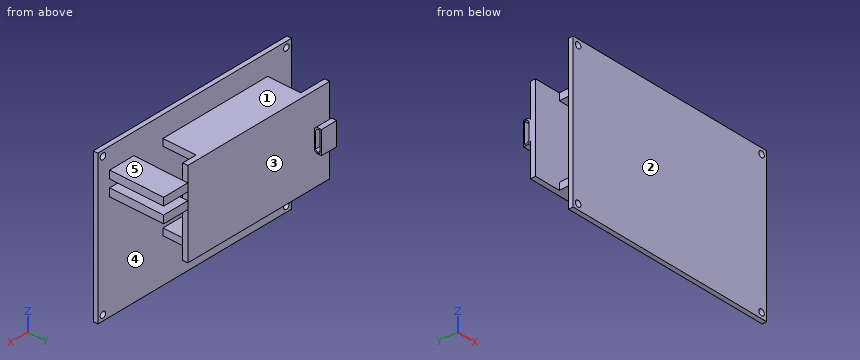
Autodesk Inventor part; units mm, degrees
ref_plane "YZ Plane" through (0, 0, 0) normal (1, 0, 0) x (0, 1, 0)
ref_plane "XZ Plane" through (0, 0, 0) normal (0, 1, 0) x (-1, 0, 0)
ref_plane "XY Plane" through (0, 0, 0) normal (0, 0, 1) x (1, 0, 0)
sketch "Sketch1" plane through (0, 0, 0) normal (0, 1, 0) x (-1, 0, 0)
  line L0 (-35, 25) -> (35, 25)
  line L1 (35, 25) -> (35, -25)
  line L2 (35, -25) -> (-35, -25)
  line L3 (-35, -25) -> (-35, 25)
  line L4 (-35, 25) -> (35, -25) construction
  line L5 (35, 25) -> (-35, -25) construction
  point P0 (0, 0)
  dimension "d0" = 70
  dimension "d1" = 50
extrude "Extrusion1" add sketch "Sketch1" along normal blind 1.5
sketch "Sketch4" plane through (0, 1.5, 0) normal (0, 1, 0) x (1, 0, 0)
  line L0 (16.25, 10.5) -> (-35, 10.5)
  line L1 (-35, 10.5) -> (-35, -18)
  line L2 (-35, -18) -> (16.25, -18)
  line L3 (16.25, -18) -> (16.25, 10.5)
  line L4 (16.25, 10.5) -> (-35, -18) construction
  line L5 (-35, 10.5) -> (16.25, -18) construction
  line L6 (-35, -25) -> (35, -25)
  line L7 (-35, 25) -> (-35, -25)
  dimension "d10" = 51.25
  dimension "d11" = 28.5
  dimension "d12" = 7
extrude "Extrusion3" add sketch "Sketch4" along normal blind 12.7
sketch "Sketch5" plane through (0, 1.5, 0) normal (0, 1, 0) x (1, 0, 0)
  line L0 (30.74, -15.4) -> (22, -15.4)
  line L1 (22, -15.4) -> (22, -18)
  line L2 (22, -18) -> (30.74, -18)
  line L3 (30.74, -18) -> (30.74, -15.4)
  line L4 (30.74, -15.4) -> (22, -18) construction
  line L5 (22, -15.4) -> (30.74, -18) construction
  line L6 (16.25, -18) -> (16.25, 10.5)
  line L7 (-35, -18) -> (16.25, -18)
  line L8 (30.74, -10.2) -> (22, -10.2)
  line L9 (22, -10.2) -> (22, -12.8)
  line L10 (22, -12.8) -> (30.74, -12.8)
  line L11 (30.74, -12.8) -> (30.74, -10.2)
  line L12 (30.74, -10.2) -> (22, -12.8) construction
  line L13 (22, -10.2) -> (30.74, -12.8) construction
  point P0 (0, 0)
  point P1 (26.37, -16.7)
  point P2 (22, -16.7)
  point P3 (26.37, -11.5)
  point P4 (22, -11.5)
  dimension "d15" = 5.75
  dimension "d16" = 8.74
  dimension "d17" = 2.6
  dimension "d18" = 8.74
  dimension "d19" = 2.6
  dimension "d20" = 2.6
extrude "Extrusion4" add sketch "Sketch5" along normal blind 18
sketch "Sketch6" plane through (-35, 0, -25) normal (-1, 0, 0) x (0, 0, 1)
  line L0 (24.91, 16.55) -> (32.59, 16.55)
  line L1 (32.59, 16.55) -> (32.59, 14.9)
  line L2 (31.89, 14.2) -> (25.61, 14.2)
  line L3 (24.91, 14.9) -> (24.91, 16.55)
  line L4 (24.91, 16.55) -> (32.59, 14.2) construction
  line L5 (32.59, 16.55) -> (24.91, 14.2) construction
  line L6 (43, 1.5) -> (50, 1.5)
  line L7 (43, 1.5) -> (43, 14.2)
  line L8 (14.5, 1.5) -> (14.5, 14.2)
  line L9 (32.18, 16.14) -> (25.32, 16.14)
  line L10 (25.32, 16.14) -> (25.32, 15.31)
  line L11 (26.02, 14.61) -> (31.48, 14.61)
  line L12 (32.18, 15.31) -> (32.18, 16.14)
  line L13 (14.5, 14.2) -> (43, 14.2)
  line L14 (25.32, 15.31) -> (26.02, 14.61)
  line L15 (32.18, 15.31) -> (31.48, 14.61)
  line L16 (32.59, 14.9) -> (31.89, 14.2)
  line L17 (24.91, 14.9) -> (25.61, 14.2)
  point P0 (25, 0)
  point P1 (28.75, 15.375)
  point P2 (25.32, 14.61)
  point P3 (32.18, 14.61)
  dimension "d24" = 2.35
  dimension "d25" = 7.68
  dimension "d26" = 14.25
  dimension "d27" = 14.25
  dimension "d28" = 0.41
  dimension "d50" = 0.7
  dimension "d51" = 0.7
  dimension "d52" = 0.7
  dimension "d53" = 0.7
  dimension "d54" = 0.7
  dimension "d55" = 0.7
  dimension "d56" = 0.7
  dimension "d57" = 0.7
extrude "Extrusion5" add sketch "Sketch6" against normal blind 5.51
sketch "Sketch8" plane through (0, 1.5, 0) normal (0, 1, 0) x (1, 0, 0)
  circle A0 centre (33.16, -23.16) radius 1
  circle A1 centre (-33.16, -23.16) radius 1
  circle A2 centre (-33.16, 23.16) radius 1
  circle A3 centre (33.16, 23.16) radius 1
  line L0 (22, -10.2) -> (30.74, -10.2)
  line L1 (30.74, -10.2) -> (30.74, -12.8)
  line L2 (30.74, -12.8) -> (22, -12.8)
  line L3 (22, -12.8) -> (22, -10.2)
  line L4 (22, -15.4) -> (30.74, -15.4)
  line L5 (30.74, -15.4) -> (30.74, -18)
  line L6 (30.74, -18) -> (22, -18)
  line L7 (22, -18) -> (22, -15.4)
  line L8 (16.25, -18) -> (-35, -18)
  line L9 (-35, -18) -> (-35, -25)
  line L10 (-35, -25) -> (35, -25)
  line L11 (35, -25) -> (35, 25)
  line L12 (35, 25) -> (-35, 25)
  line L13 (-35, 25) -> (-35, 10.5)
  line L14 (-35, 10.5) -> (16.25, 10.5)
  line L15 (16.25, 10.5) -> (16.25, -18)
  point P0 (0, 0)
  dimension "d33" = 2
  dimension "d34" = 2
  dimension "d35" = 2
  dimension "d36" = 2
  dimension "d37" = 1.84
  dimension "d38" = 1.84
  dimension "d39" = 1.84
  dimension "d40" = 1.84
  dimension "d41" = 1.84
  dimension "d42" = 1.84
  dimension "d43" = 1.84
  dimension "d44" = 1.84
extrude "Extrusion7" cut sketch "Sketch8" against normal blind 10 contours A0 | A1 | A2 | A3
sketch "Sketch9" plane through (-35, 0, -25) normal (-1, 0, 0) x (0, 0, 1)
  line L0 (14.5, 1.5) -> (14.5, 14.2) construction
  line L1 (43, 1.5) -> (43, 19.5) construction
  line L2 (14.5, 14.2) -> (43, 14.2) construction
  line L3 (43, 14.2) -> (43, 1.5) construction
  line L4 (43, 1.5) -> (14.5, 1.5) construction
  line L5 (14.5, 1.5) -> (14.5, 14.2) construction
  line L6 (40.7, 12.5) -> (16.8, 12.5)
  line L7 (16.8, 12.5) -> (16.8, 1.5)
  line L8 (40.7, 1.5) -> (40.7, 12.5)
  line L9 (16.8, 1.5) -> (40.7, 1.5)
  point P0 (25, 0)
  point P1 (14.5, 7.85)
  dimension "d47" = 1.7
  dimension "d64" = 2.3
  dimension "d65" = 2.3
extrude "Extrusion8" cut sketch "Sketch9" against normal up to next
sketch "Sketch10" plane through (16.25, 1.5, -10.5) normal (0, 0, -1) x (-1, 0, 0)
  line L0 (51.25, 0) -> (0, 0)
  line L1 (51.25, 0) -> (51.25, 12.7)
  line L2 (0, 12.7) -> (51.25, 12.7)
  line L3 (0, 0) -> (0, 12.7)
  line L4 (51.25, 11) -> (0, 11)
  line L5 (51.25, 0) -> (0, 0)
  line L6 (51.25, 11) -> (42.65, 11)
  line L7 (42.65, 11) -> (42.65, 0)
  line L8 (42.65, 0) -> (51.25, 0)
  line L9 (51.25, 0) -> (51.25, 11)
  point P0 (16.25, -1.5)
  point P1 (42.65, 0)
  dimension "d58" = 8.6
extrude "Extrusion9" cut sketch "Sketch10" against normal through all contours L0 L7 L4 L1
sketch "Sketch11" plane through (16.25, 14.2, -10.5) normal (0, 0, -1) x (-1, 0, 0)
  line L0 (42.65, -1.7) -> (0, -1.7)
  line L1 (42.65, -12.7) -> (0, -12.7)
  line L2 (0, -1.7) -> (4.8, -1.7)
  line L3 (4.8, -1.7) -> (4.8, -12.7)
  line L4 (4.8, -12.7) -> (0, -12.7)
  line L5 (0, -12.7) -> (0, -1.7)
  point P0 (16.25, -14.2)
  point P1 (0, -12.7)
  point P2 (4.8, -1.7)
  dimension "d61" = 4.8
extrude "Extrusion10" cut sketch "Sketch11" against normal through all
equation "\"d54\" = d50"
equation "\"d55\" = d54"
equation "\"d56\" = d50"
equation "\"d57\" = d56"
equation "\"d38\" = d37"
equation "\"d39\" = d37"
equation "\"d40\" = d37"
equation "\"d41\" = d37"
equation "\"d42\" = d37"
equation "\"d43\" = d37"
equation "\"d44\" = d37"
equation "\"d65\" = d64"
properties part number "PCBModel"
Work out the finished part from the listing and answer in its coordinate system (mm). Face numbers are marked on the shaded views. A direction names the side the tool comes from. Round coordinates to 2 decimals unless told otherwise and drop trailing zeros. Write each loop counter-clockwise with the first axis right and the second up, starting at its lowest first coordinate (ties: lowest second). Pieces come first, ordered by that corner, then holes. Notation, with made-up numbers: (-5.5, -16) -> (16.5, -16) arc R8 cw to (16.5, -10) -> close; hole circle Ø1 at (62.25, 89). An arc over 180 degrees is marked (long way). Write each question's results on one line, items separated by ' | '.
Q1. Section D-D, the plane z = 4.5 is taken. Write down the section's boundary in (x, y).
Data:
outline: (-35, 0) -> (35, 0) -> (35, 1.5) -> (-35, 1.5) -> close; (-35, 12.5) -> (16.25, 12.5) -> (16.25, 14.2) -> (-29.49, 14.2) -> (-29.49, 14.61) -> (-35, 14.61) -> close; (-35, 16.14) -> (-29.49, 16.14) -> (-29.49, 16.55) -> (-35, 16.55) -> close
Q2. Flat-ended cylindrical pins translate along their axes: P1, Ø0.5, axis at x = -31, y = 15.5, coming from the -Z side; P2, Ø1.8, axis at x = -31, y = 16, coming from the +Z side; P3, Ø10, axis at x = 16, y = 15.5, coming from the -Z side. Find the tip coordinate at first contact, or state that the pin passes through.
Data:
P1: z = -0.09 | P2: z = 7.59 | P3: z = -10.5
Q3. Section B-B, the plane x = -33.16 is taken. Write down the section's boundary in (y, z), then the cut area to 3 significant figures.
Data:
outline: (0, -25) -> (1.5, -25) -> (1.5, -24.16) -> (0, -24.16) -> close; (0, -22.16) -> (1.5, -22.16) -> (1.5, 22.16) -> (0, 22.16) -> close; (0, 24.16) -> (1.5, 24.16) -> (1.5, 25) -> (0, 25) -> close; (12.5, -10.5) -> (14.2, -10.5) -> (14.2, 0.61) -> (14.9, -0.09) -> (16.55, -0.09) -> (16.55, 7.59) -> (14.9, 7.59) -> (14.2, 6.89) -> (14.2, 18) -> (12.5, 18) -> close; hole (14.61, 1.02) -> (15.31, 0.32) -> (16.14, 0.32) -> (16.14, 7.18) -> (15.31, 7.18) -> (14.61, 6.48) -> close | area: 125 mm^2
Q4. Section C-C, the plane y = 7.75 is taken. Write down the section's boundary in (x, z), then the cut area to 3 significant figures.
Data:
outline: (-26.4, -10.5) -> (11.45, -10.5) -> (11.45, -8.2) -> (-26.4, -8.2) -> close; (-26.4, 15.7) -> (11.45, 15.7) -> (11.45, 18) -> (-26.4, 18) -> close; (22, 10.2) -> (30.74, 10.2) -> (30.74, 12.8) -> (22, 12.8) -> close; (22, 15.4) -> (30.74, 15.4) -> (30.74, 18) -> (22, 18) -> close | area: 220 mm^2
Q5. Straight lines are drawn through the part: line 1 along X through (y, z) = (1, -23.16); line 2 along Z through (x, y) = (-33.16, 1.05); line 3 along X through (y, z) = (3.25, 17). For each, find the intervals that lie inside material, in ascending order. Write a range as [from, to].
Data:
line 1: [-35, -34.16], [-32.16, 32.16], [34.16, 35] | line 2: [-25, -24.16], [-22.16, 22.16], [24.16, 25] | line 3: [-26.4, 11.45], [22, 30.74]
Q6. Determine the mould class of the marked faces 3, 4 and 5 for opening direction Z: released by +Z, released by -Z, zero draft, split by the parting line, or undercut.
Data:
face 3: zero draft | face 4: undercut | face 5: released by +Z
Q7. Section A-A, the plane z = -4 is taken. Write down the section's boundary in (x, y), then the cut area to 3 significant figures.
Data:
outline: (-35, 0) -> (35, 0) -> (35, 1.5) -> (-35, 1.5) -> close; (-35, 12.5) -> (16.25, 12.5) -> (16.25, 14.2) -> (-35, 14.2) -> close | area: 192 mm^2
Q8. Which of the six approach directions +Z, -Z, +X, -X, +Y, -Y give full straight-line access (tool end or side, diameter ignored) to the marked faces 1 and 2?
Data:
face 1: +Z, +X, -X, +Y | face 2: +Z, -Z, +X, -X, -Y
